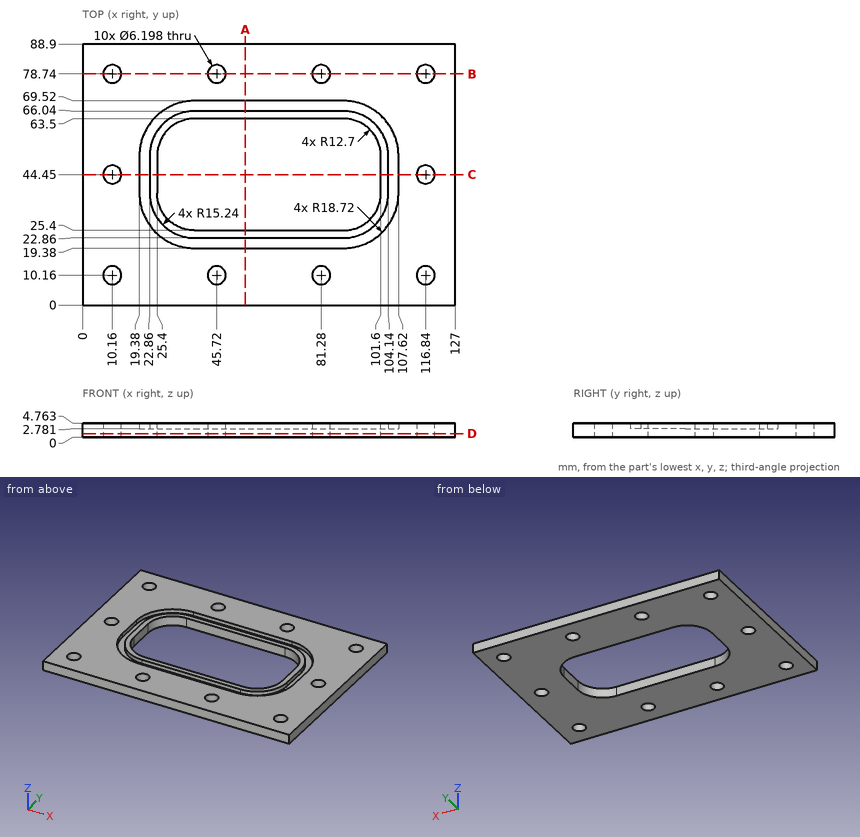
Source: three-view drawing plus pictorial views. Frame: mm from the lowest corner of the part. Round coordinates to 2 decimals unless told otherwise and drop trailing zeros. Loops run counter-clockwise (first coordinate to the right, second up) from the corner with the lowest first, then second, coordinate; pieces in that order, holes last.
Q1. Section A-A, the plane x = 55.5. Return loops of the section in (y, z).
Q2. Section C-C, the plane y = 44.45. Return loops of the section in (x, z).
Q3. Section D-D, the plane z = 1.15. State how many separate pieces and enclosed holes the cut face has, plus the area to 3 significant figures.
Q4. Section B-B, the plane y = 78.74. Return loops of the section in (x, z), plus the area to 3 significant figures.
Q5. Ray query, line 1 (Y direction, x = 51, z = 4.3); line 2 (Y direction, x = 10.16, z = 2.9); line 3 (Y direction, x = 45.72, z = 3.4). Return the intervals inside material, ascending.
Solutions:
1. outline: (0, 0) - (25.4, 0) - (25.4, 4.76) - (22.86, 4.76) - (22.86, 2.78) - (19.38, 2.78) - (19.38, 4.76) - (0, 4.76) - close; (63.5, 0) - (88.9, 0) - (88.9, 4.76) - (69.52, 4.76) - (69.52, 2.78) - (66.04, 2.78) - (66.04, 4.76) - (63.5, 4.76) - close
2. outline: (0, 0) - (7.06, 0) - (7.06, 4.76) - (0, 4.76) - close; (13.26, 0) - (25.4, 0) - (25.4, 4.76) - (22.86, 4.76) - (22.86, 2.78) - (19.38, 2.78) - (19.38, 4.76) - (13.26, 4.76) - close; (101.6, 0) - (113.74, 0) - (113.74, 4.76) - (107.62, 4.76) - (107.62, 2.78) - (104.14, 2.78) - (104.14, 4.76) - (101.6, 4.76) - close; (119.94, 0) - (127, 0) - (127, 4.76) - (119.94, 4.76) - close
3. separate pieces: 1
3. enclosed holes: 11
3. area: 8,220 mm2
4. outline: (0, 0) - (7.06, 0) - (7.06, 4.76) - (0, 4.76) - close; (13.26, 0) - (42.62, 0) - (42.62, 4.76) - (13.26, 4.76) - close; (48.82, 0) - (78.18, 0) - (78.18, 4.76) - (48.82, 4.76) - close; (84.38, 0) - (113.74, 0) - (113.74, 4.76) - (84.38, 4.76) - close; (119.94, 0) - (127, 0) - (127, 4.76) - (119.94, 4.76) - close
4. area: 487 mm2
5. line 1: y = 0 to 19.38, 22.86 to 25.4, 63.5 to 66.04, 69.52 to 88.9
5. line 2: y = 0 to 7.06, 13.26 to 41.35, 47.55 to 75.64, 81.84 to 88.9
5. line 3: y = 0 to 7.06, 13.26 to 19.38, 22.86 to 25.4, 63.5 to 66.04, 69.52 to 75.64, 81.84 to 88.9
